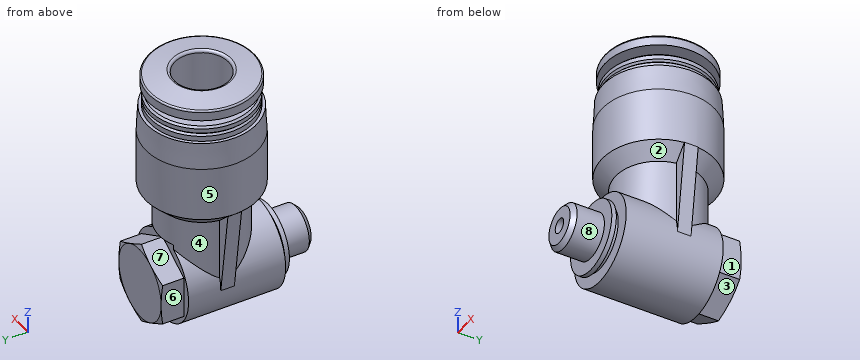
from build123d import *

# Parameters (mm, degrees)
LINEAR_AUSTRAGEN1_DEPTH      = 0.75
LINEAR_AUSTRAGEN1_DEPTH_BACK = 0.75
SKIZZE5_W                    = 16
SKIZZE5_H                    = 16
LINEAR_AUSTRAGEN2_DEPTH      = 2.5
SKIZZE6_W                    = 0.8
SKIZZE6_H                    = 10.9


with BuildPart() as part:
    # Skizze1 → Rotation1 (revolve)
    with BuildSketch(Plane(origin=(0, 0, 0), x_dir=(0, 0, -1), z_dir=(1, 0, 0))):
        Polygon((0, 6.8), (4, 6.8), (4.9, 6.558845727), (4.9, -6.4), (3.4, -6.4), (3.4, -6.9), (3.9, -6.9), (3.9, -7.4), (2.5, -7.4), (2.5, -10.4095), (2.0095, -10.9), (0, -10.9), align=None)
    revolve(axis=Axis((0, -10.9, 0), (0, 1, 0)))

    # Skizze2 → Rotation2 (revolve)
    with BuildSketch(Plane(origin=(0, 0, 0), x_dir=(0, 0, -1), z_dir=(1, 0, 0))):
        with BuildLine():
            Line((0, -4.75), (-8.35, -4.75))
            Line((-8.35, -4.75), (-9.85, -6.25))
            Line((-9.85, -6.25), (-15.9, -6.25))
            Line((-15.9, -6.25), (-18.9, -6.092776662))
            Line((-18.9, -6.092776662), (-18.9, -5.75))
            Line((-18.9, -5.75), (-19.5, -5.75))
            Line((-19.5, -5.75), (-19.7, -5.55))
            Line((-19.7, -5.55), (-19.9, -5.75))
            Line((-19.9, -5.75), (-20.387867966, -5.75))
            Line((-20.387867966, -5.75), (-20.6, -5.537867966))
            Line((-20.6, -5.537867966), (-20.6, -4.05))
            Line((-20.6, -4.05), (-21.3, -4.05))
            ThreePointArc((-21.3, -4.05), (-21.441421356, -4.108578644), (-21.5, -4.25))
            Line((-21.5, -4.25), (-21.5, -5.9))
            Line((-21.5, -5.9), (-22.473729924, -5.9))
            ThreePointArc((-22.473729924, -5.9), (-22.602287446, -5.853208889), (-22.670691475, -5.734729636))
            Line((-22.670691475, -5.734729636), (-23.1, -3.3))
            Line((-23.1, -3.3), (-23.1, 0))
            Line((-23.1, 0), (4.75, 0))
            ThreePointArc((4.75, 0), (3.358757211, -3.358757211), (0, -4.75))
        make_face()
    revolve(axis=Axis((0, 0, 23.1), (0, 0, -1)))

    # Skizze4 → Linear austragen1 (add, two sides)
    with BuildSketch(Plane(origin=(0, 0, 0), x_dir=(1, 0, 0), z_dir=(0, 1, 0))) as linear_austragen1_sk:
        Polygon((-6.25, -9.85), (6.25, -9.85), (4.9, 0), (-4.9, 0), align=None)
    extrude(amount=LINEAR_AUSTRAGEN1_DEPTH)
    extrude(linear_austragen1_sk.sketch, amount=-LINEAR_AUSTRAGEN1_DEPTH_BACK)

    # Skizze5 → Linear austragen2 (cut)
    with BuildSketch(Plane(origin=(0, 4.3, 0), x_dir=(-1, 0, 0), z_dir=(0, 1, 0))):
        with Locations((0, -3)):
            Rectangle(SKIZZE5_W, SKIZZE5_H)
        Polygon((4, 2.309401077), (0, 4.618802154), (-4, 2.309401077), (-4, -2.309401077), (0, -4.618802154), (4, -2.309401077), align=None, mode=Mode.SUBTRACT)
    extrude(amount=LINEAR_AUSTRAGEN2_DEPTH, mode=Mode.SUBTRACT)

    # Skizze6 → Schnitt-Rotation1 (revolve, cut)
    with BuildSketch(Plane(origin=(0, 0, 0), x_dir=(0, 0, -1), z_dir=(1, 0, 0))):
        with Locations((0.4, -5.45)):
            Rectangle(SKIZZE6_W, SKIZZE6_H)
    revolve(axis=Axis((0, -10.9, 0), (0, 1, 0)), mode=Mode.SUBTRACT)

    # Skizze3 → Schnitt-Rotation2 (revolve, cut)
    with BuildSketch(Plane(origin=(0, 0, 0), x_dir=(0, 0, -1), z_dir=(1, 0, 0))):
        with BuildLine():
            Line((0, -0.8), (-6.1, -0.8))
            Line((-6.1, -0.8), (-6.1, -3))
            Line((-6.1, -3), (-22.8, -3))
            ThreePointArc((-22.8, -3), (-23.012132034, -3.087867966), (-23.1, -3.3))
            Line((-23.1, -3.3), (-23.1, 0))
            Line((-23.1, 0), (0.8, 0))
            ThreePointArc((0.8, 0), (0.565685425, -0.565685425), (0, -0.8))
        make_face()
    revolve(axis=Axis((0, 0, 23.1), (0, 0, -1)), mode=Mode.SUBTRACT)


solid = part.part
For this review, take the finished solid that the model builds, in its own axes (mm). Face numbers are marked on the shaded views. A direction names the side the tool comes from. Round coordinates to 2 decimals unless told otherwise and drop trailing zeros. Write each loop counter-clockwise with the first axis right and the second up, starting at its lowest first coordinate (ties: lowest second). Pieces come first, ordered by that corner, then holes. Notation, with made-up numbers: M -25.75,32 L 13.25,32 A19 cw 13.25,40 Z; hole C 4,-9.5 d8. An arc over 180 degrees is marked long. Write item = value, one per line. Start each with the question number.
(1) The part is to be moulded in two halves that separate along Z. For the marked faces 1, 2 and 3, say which applies: +Z half, -Z half, draft (parallel to the pull), parting line (faces both ways), or undercut.
(2) Clearance check with flat-ended pins moving along their axes: pin 1 Ø10 at (y, z) = (-1.5, 19.5) entering from +X; pin 2 Ø0.7 at (y, z) = (5.5, 1) entering from -X; pin 3 Ø3 at (x, z) = (2, 19.5) entering from +Y; pin 4 Ø2 at (x, z) = (-1, 14.5) entering from -Y. State where each tip first meets the part, or that it passes through.
(3) We need section A-A (z = 16.5). Give the boundary of the cut face in (x, y).
(4) For the marked faces 4, 5, 6, 7 and 8, list the 3-axis set-ups (+Z, -Z, +X, -X, +Y, -Y) from which the entire face can be reached by the end or side of a thin tool; tool diameter is ignored.
(5) For line 1 along Y through (x, z) = (0, 14.75); line 2 along Z through (x, y) = (1.5, 5.25); line 3 along Y through (x, z) = (0, 19.5), list the stretches that pass through material, from the lowest coordinate up.
(6) We need section B-B (y = 5.25). Give the number of separate pieces and of enclosed holes in the cut face, then the cut area to 3 significant figures.
Results found:
q1.face_1 = draft
q1.face_2 = undercut
q1.face_3 = -Z half
q2.pin_1 = 6.25
q2.pin_2 = -4
q2.pin_3 = 6.06
q2.pin_4 = -6.25
q3.outline = C 0,0 d12.44; hole C 0,0 d6
q4.face_4 = +Y
q4.face_5 = +Z
q4.face_6 = -Z, -X, +Y
q4.face_7 = -X, +Y
q4.face_8 = -Y
q5.line_1 = -6.25 to -3, 3 to 6.25
q5.line_2 = -3.75 to 3.75, 9.06 to 20.6, 21.5 to 22.72
q5.line_3 = -5.75 to -3, 3 to 5.75
q6.separate_pieces = 3
q6.enclosed_holes = 0
q6.area = 135 mm²
